For this review, take the finished solid that the model builds, in its own axes (mm). A direction names the side the tool comes from. Coordinates: 2 decimals unless noted, no trailing zeros. Write each loop counter-clockwise with the first axis right and the second up, starting at its lowest first coordinate (ties: lowest second). Pieces come first, ordered by that corner, then holes.
```python
from build123d import *

# Parameters (mm, degrees)
SKETCH_1_W          = 35
SKETCH_1_H          = 43.5
EXTRUDE_1_DEPTH     = 20
SKETCH_2_W          = 20
SKETCH_2_H          = 5
EXTRUDE_2_DEPTH     = 10
SKETCH_3_W          = 20
SKETCH_3_H          = 5
EXTRUDE_3_DEPTH     = 10
SKETCH_4_R          = 1.5
CUT_EXTRUDE_2_DEPTH = 5
SKETCH_5_R          = 13
CUT_EXTRUDE_3_DEPTH = 20


with BuildPart() as part:
    # Эскиз1 → Бобышка-Вытянуть1 (new body)
    with BuildSketch(Plane.XY):
        Rectangle(SKETCH_1_W, SKETCH_1_H)
    extrude(amount=EXTRUDE_1_DEPTH)

    # Эскиз2 → Бобышка-Вытянуть2 (add)
    with BuildSketch(Plane(origin=(17.5, 0, 0), x_dir=(0, 0, -1), z_dir=(1, 0, 0))):
        with Locations((-10, -19.25)):
            Rectangle(SKETCH_2_W, SKETCH_2_H)
    extrude(amount=EXTRUDE_2_DEPTH)

    # Эскиз3 → Бобышка-Вытянуть3 (add)
    with BuildSketch(Plane.ZY.offset(17.5)):
        with Locations((10, -19.25)):
            Rectangle(SKETCH_3_W, SKETCH_3_H)
    extrude(amount=EXTRUDE_3_DEPTH)

    # Эскиз4 → Вырез-Вытянуть2 (cut)
    with BuildSketch(Plane(origin=(0, -16.75, 0), x_dir=(1, 0, 0), z_dir=(0, 1, 0))):
        with Locations((-22.5, -16)):
            Circle(SKETCH_4_R)
        with Locations((-22.5, -4)):
            Circle(SKETCH_4_R)
        with Locations((22.5, -16)):
            Circle(SKETCH_4_R)
        with Locations((22.5, -4)):
            Circle(SKETCH_4_R)
    extrude(amount=-CUT_EXTRUDE_2_DEPTH, mode=Mode.SUBTRACT)

    # Эскиз5 → Вырез-Вытянуть3 (cut)
    with BuildSketch(Plane(origin=(0, 0, 0), x_dir=(-1, 0, 0), z_dir=(0, 0, -1))):
        with Locations((0, 8.25)):
            Circle(SKETCH_5_R)
    extrude(amount=-CUT_EXTRUDE_3_DEPTH, mode=Mode.SUBTRACT)


solid = part.part
```
Q1. Add section D-D (x = 0). State the section outline as (y, z) points, then the cut area to 3 significant figures.
Ans:
outline: (-21.75, 0) - (-4.75, 0) - (-4.75, 20) - (-21.75, 20) - close; (21.25, 0) - (21.75, 0) - (21.75, 20) - (21.25, 20) - close
area: 350 mm2
Q2. Add section C-C (y = 8.25). State the section outline as (x, z) points, then the cut area to 3 significant figures.
Ans:
outline: (-17.5, 0) - (-13, 0) - (-13, 20) - (-17.5, 20) - close; (13, 0) - (17.5, 0) - (17.5, 20) - (13, 20) - close
area: 180 mm2
Q3. Clearance check with flat-ended pins moving along their axes: pin 1 Ø3.5 at (x, z) = (-22.5, 4) entering from +Y; pin 2 Ø10 at (y, z) = (9.5, 7.5) entering from -X; pin 3 Ø6 at (y, z) = (10.5, 12) entering from +X. State where each tip first meets the part, or that it passes through.
Ans:
pin 1: stops at y = -16.75
pin 2: stops at x = -17.5
pin 3: stops at x = 17.5
Q4. For probe 1 along X at (y, z) = (-19.6, 16); probe 2 along Z at (x, y) = (-22.5, -18.1); probe 3 along X at (y, z) = (-17, 15.25), list the stretches that pass through material, from the lowest coordinate up.
Ans:
probe 1: x = -27.5 to -24, -21 to 21, 24 to 27.5
probe 2: z = 0 to 2.5, 5.5 to 14.5, 17.5 to 20
probe 3: x = -27.5 to -23.8, -21.2 to 21.2, 23.8 to 27.5
Q5. Draft analysis for pull direction Y (two halves, no side actions). For faces 1 (the cylindrical face through (10.316, 0.34, 9.86)), 2 (the flat face through (0, -10, 20)), 3 (the flat face through (22, -16.75, 10)), state which applies: +Y half, -Y half, draft (parallel to the pull), parting line (faces both ways), or undercut.
Ans:
face 1: undercut
face 2: draft
face 3: +Y half
Q6. Tool access review of faces 4 (the flat face through (17.5, 2, 10)), 5 (the flat face through (-22, -16.75, 10)), 6 (the flat face through (0, -10, 0)): name each direction out of +Z, -Z, +X, -X, +Y, -Y from which nothing blocks a thin tool from reaching the whole face with its end or side.
Ans:
face 4: +Z, -Z, +X, +Y
face 5: +Z, -Z, -X, +Y
face 6: -Z, +X, -X, +Y, -Y
Q7. Add section B-B (x = -22.5). State the section outline as (y, z) points.
Ans:
outline: (-21.75, 0) - (-16.75, 0) - (-16.75, 2.5) - (-21.75, 2.5) - close; (-21.75, 5.5) - (-16.75, 5.5) - (-16.75, 14.5) - (-21.75, 14.5) - close; (-21.75, 17.5) - (-16.75, 17.5) - (-16.75, 20) - (-21.75, 20) - close
Q8. Add section A-A (z = 4). State the section outline as (x, y) points, then the cut area to 3 significant figures.
Ans:
outline: (-27.5, -21.75) - (-24, -21.75) - (-24, -16.75) - (-27.5, -16.75) - close; (-21, -21.75) - (21, -21.75) - (21, -16.75) - (17.5, -16.75) - (17.5, 21.75) - (-17.5, 21.75) - (-17.5, -16.75) - (-21, -16.75) - close; (24, -21.75) - (27.5, -21.75) - (27.5, -16.75) - (24, -16.75) - close; hole circle Ø26 at (0, 8.25)
area: 1,060 mm2
